CAD build for the part. Positions are in the model's coordinates, mm. A direction names the side the tool comes from. Coordinates: 2 decimals unless noted, no trailing zeros. Loops run counter-clockwise (first coordinate to the right, second up) from the corner with the lowest first, then second, coordinate; pieces in that order, holes last. Notation, with made-up numbers: (20, 82.5) -> (39, 82.5) arc R23 cw to (39, 106.5) -> close; hole circle Ø11 at (68, 63). An arc over 180 degrees is marked (long way). Write item = value, one per line. Start each with the question number.
(1) Band-saw the part on A-A (y = 80). Write the cut outline in (x, z), and give its area (3 significant figures).
(2) Tool access for faces 5 (the face through (-28, 80, -3)), 6 (the face through (-114.937, 79, -3)), 7 (the face through (92, 10.635, -2)): list every direction of +Z, -Z, +X, -X, +Y, -Y with a clear straight run to the whole face (end or side of a thin tool).
(3) Drill centre lines: line 1 (Y direction, x = -46, z = -1.1); line 2 (Y direction, x = -13, z = -2.75); line 3 (X direction, y = 102, z = -1.9). Where is each one in solid material? Low to high. Write a range as from..to.
(4) Band-saw the part on B-B (z = -4.1). Count the separate pieces of the cut face and the enclosed holes in it, and give its area (3 significant figures).
(5) Band-saw the part on D-D (y = 160.5). Write the cut outline in (x, z).
(6) Flat gauge pins, fed straight in: P1, Ø3, axis at x = -46, y = 64.7, coming from the -Z side; P2, Ø6.5, axis at x = -46, y = 96.7, coming from the +Z side; P3, Ø2, axis at y = 44, z = -1, coming from the +X side; P4, Ø2.5, axis at x = 92.5, z = -3.5, coming from the +Y side. Where does each tip first touch, or does it go through?
(7) Pull direction Y, two halves, no side cores. Call faces 1 (the face through (-92.253, -8.116, -2.535)), 2 (the face through (72.542, 52.695, -2.535)), 3 (the face through (-30, 82, 0)), 4 (the face through (-39, 180.635, -2)): +Y half, -Y half, draft (parallel to the pull), parting line (faces both ways), or undercut.
(8) Band-saw the part on C-C (x = 72). Write the cut outline in (y, z), and give its area (3 significant figures).
```python
from build123d import *

# Parameters (mm, degrees)
BOSS_EXTRUDE1_DEPTH = 5
SKETCH2_R           = 2.5
SKETCH2_W           = 35
SKETCH2_H           = 75
CUT_EXTRUDE1_DEPTH  = 10
SKETCH4_R           = 2
CUT_EXTRUDE3_DEPTH  = 10
SKETCH5_R           = 2.5
CUT_EXTRUDE4_DEPTH  = 10
SKETCH6_W           = 242.754098284
SKETCH6_H           = 200
CUT_EXTRUDE5_DEPTH  = 10


with BuildPart() as part:
    # Sketch1 → Boss-Extrude1 (new body)
    with BuildSketch(Plane.XY):
        with BuildLine():
            Line((77, 150.635083269), (106.477021815, 150.635083269))
            ThreePointArc((106.477021815, 150.635083269), (73.792570992, 172.830527842), (35.06273753, 180.635083269))
            Line((35.06273753, 180.635083269), (-264.93726247, 180.635083269))
            ThreePointArc((-264.93726247, 180.635083269), (-303.667095932, 172.830527842), (-336.351546756, 150.635083269))
            Line((-336.351546756, 150.635083269), (-306.874524941, 150.635083269))
            Line((-306.874524941, 150.635083269), (-306.874524941, 10.635083269))
            Line((-306.874524941, 10.635083269), (-336.351546756, 10.635083269))
            ThreePointArc((-336.351546756, 10.635083269), (-303.667095932, -11.560361304), (-264.93726247, -19.364916731))
            Line((-264.93726247, -19.364916731), (35.06273753, -19.364916731))
            ThreePointArc((35.06273753, -19.364916731), (73.792570992, -11.560361304), (106.477021815, 10.635083269))
            Line((106.477021815, 10.635083269), (77, 10.635083269))
            Line((77, 10.635083269), (77, 150.635083269))
        make_face()
    extrude(amount=-BOSS_EXTRUDE1_DEPTH)

    # Sketch2 → Cut-Extrude1 (cut)
    with BuildSketch(Plane(origin=(0, 0, -5), x_dir=(-1, 0, 0), z_dir=(0, 0, -1))):
        with Locations((301.874524941, 106.135083269)):
            Circle(SKETCH2_R)
        with Locations(Location((301.874524941, 55.135083269, 0), (0, 0, 180))):
            Circle(SKETCH2_R)
        with Locations((-72, 55.135083269)):
            Circle(SKETCH2_R)
        with Locations(Location((-72, 106.135083269, 0), (0, 0, 180))):
            Circle(SKETCH2_R)
        with Locations((219.374524941, 80.635083269)):
            Rectangle(SKETCH2_W, SKETCH2_H)
        with Locations((10.5, 80.635083269)):
            Rectangle(SKETCH2_W, SKETCH2_H)
    extrude(amount=-CUT_EXTRUDE1_DEPTH, mode=Mode.SUBTRACT)

    # Sketch4 → Cut-Extrude3 (cut)
    with BuildSketch(Plane(origin=(0, 0, -5), x_dir=(-1, 0, 0), z_dir=(0, 0, -1))):
        with Locations((46, 64.695083269)):
            Circle(SKETCH4_R)
        with Locations((46, 96.695083269)):
            Circle(SKETCH4_R)
        with Locations((78, 64.695083269)):
            Circle(SKETCH4_R)
        with Locations((78, 96.695083269)):
            Circle(SKETCH4_R)
        with Locations(Location((151.874524941, 64.695083269, 0), (0, 0, 180))):
            Circle(SKETCH4_R)
        with Locations(Location((183.874524941, 64.695083269, 0), (0, 0, 180))):
            Circle(SKETCH4_R)
        with Locations(Location((183.874524941, 96.695083269, 0), (0, 0, 180))):
            Circle(SKETCH4_R)
        with Locations(Location((151.874524941, 96.695083269, 0), (0, 0, 180))):
            Circle(SKETCH4_R)
    extrude(amount=-CUT_EXTRUDE3_DEPTH, mode=Mode.SUBTRACT)

    # Sketch5 → Cut-Extrude4 (cut)
    with BuildSketch(Plane(origin=(0, 0, -5), x_dir=(-1, 0, 0), z_dir=(0, 0, -1))):
        with Locations((94.63726247, 168.635083269)):
            Circle(SKETCH5_R)
        with Locations((135.23726247, 168.635083269)):
            Circle(SKETCH5_R)
        with Locations(Location((94.63726247, -7.364916731, 0), (0, 0, 180))):
            Circle(SKETCH5_R)
        with Locations(Location((135.23726247, -7.364916731, 0), (0, 0, 180))):
            Circle(SKETCH5_R)
    extrude(amount=-CUT_EXTRUDE4_DEPTH, mode=Mode.SUBTRACT)

    # Sketch6 → Cut-Extrude5 (cut)
    with BuildSketch(Plane(origin=(0, 0, -5), x_dir=(-1, 0, 0), z_dir=(0, 0, -1))):
        with Locations((236.314311612, 80.635083269)):
            Rectangle(SKETCH6_W, SKETCH6_H)
    extrude(amount=-CUT_EXTRUDE5_DEPTH, mode=Mode.SUBTRACT)


solid = part.part
```
Findings below:
q1.outline = (-114.94, -5) -> (-28, -5) -> (-28, 0) -> (-114.94, 0) -> close; (7, -5) -> (77, -5) -> (77, 0) -> (7, 0) -> close
q1.area = 785 mm²
q2.face_5 = +Z, -Z
q2.face_6 = +Z, -Z, -X, +Y, -Y
q2.face_7 = +Z, -Z, +X
q3.line_1 = -19.36..62.7, 66.7..94.7, 98.7..180.64
q3.line_2 = -19.36..43.14, 118.14..180.64
q3.line_3 = -114.94..-28, 7..77
q4.separate_pieces = 1
q4.enclosed_holes = 9
q4.area = 36,100 mm²
q5.outline = (-114.94, -5) -> (95.24, -5) -> (95.24, 0) -> (-114.94, 0) -> close
q6.P1 = through
q6.P2 = 0
q6.P3 = 77
q6.P4 = 163.36
q7.face_1 = undercut
q7.face_2 = undercut
q7.face_3 = draft
q7.face_4 = +Y half
q8.outline = (-12.29, -5) -> (52.64, -5) -> (52.64, 0) -> (-12.29, 0) -> close; (57.64, -5) -> (103.64, -5) -> (103.64, 0) -> (57.64, 0) -> close; (108.64, -5) -> (173.56, -5) -> (173.56, 0) -> (108.64, 0) -> close
q8.area = 879 mm²
